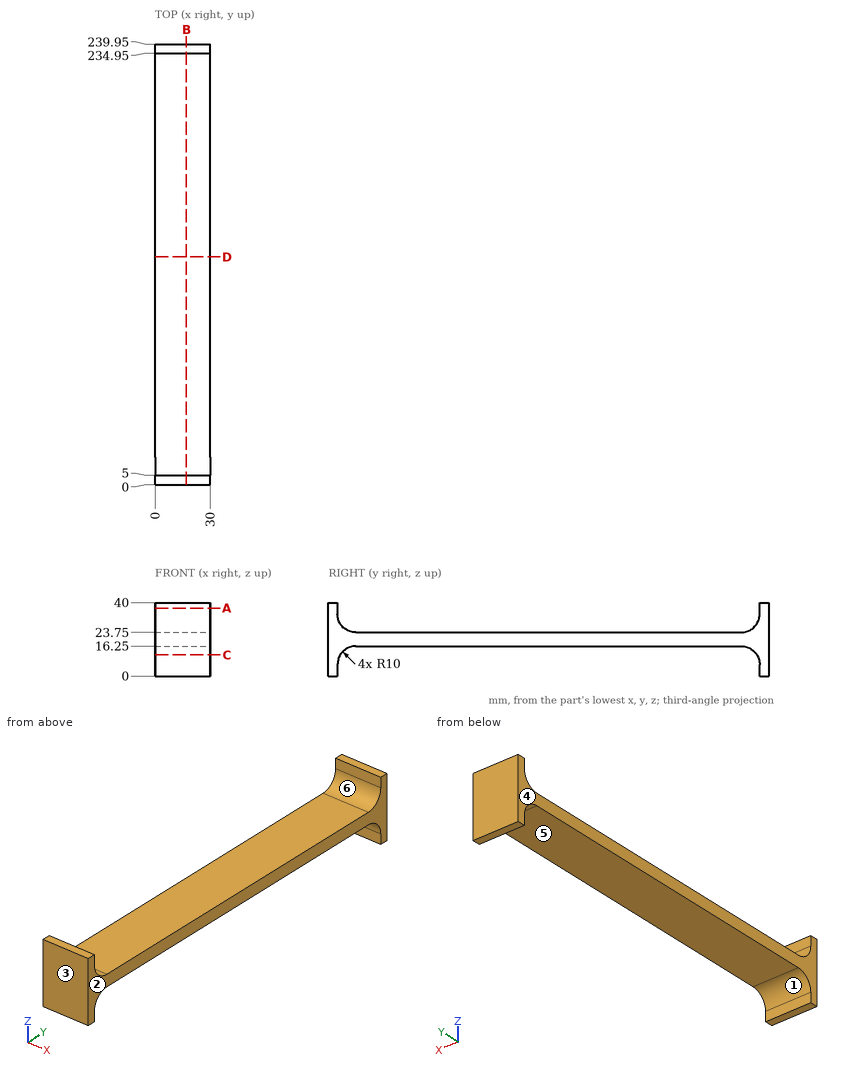
Study the drawing (mm; zero at the part's minimum x, y, z) and answer. A direction names the side the tool comes from. Coordinates: 2 decimals unless noted, no trailing zeros. Write each loop counter-clockwise with the first axis right and the second up, starting at its lowest first coordinate (ties: lowest second). Pieces come first, ordered by that corner, then holes.
Q1. Section B-B, the plane x = 17 is taken. Write down the section's boundary in (y, z), then the cut area to 3 significant figures.
Returned:
outline: (0, 0) - (5, 0) - (5, 6.25) arc R10 cw to (15, 16.25) - (224.95, 16.25) arc R10 cw to (234.95, 6.25) - (234.95, 0) - (239.95, 0) - (239.95, 40) - (234.95, 40) - (234.95, 33.75) arc R10 cw to (224.95, 23.75) - (15, 23.75) arc R10 cw to (5, 33.75) - (5, 40) - (0, 40) - close
area: 2,210 mm2
Q2. Section A-A, the plane z = 37 is taken. Write down the section's boundary in (x, y), then the cut area to 3 significant figures.
Returned:
outline: (0, 0) - (30, 0) - (30, 5) - (0, 5) - close; (0, 234.95) - (30, 234.95) - (30, 239.95) - (0, 239.95) - close
area: 300 mm2
Q3. Find the intervals of material crossed by line 1 along Y through (x, z) = (8, 36.5); line 2 along Y through (x, z) = (7.5, 7); line 3 along Z through (x, y) = (17, 168.5), in increasing order.
Returned:
line 1: y = 0 to 5, 234.95 to 239.95
line 2: y = 0 to 5.03, 234.92 to 239.95
line 3: z = 16.25 to 23.75
Q4. Which of the six approach directions +Z, -Z, +X, -X, +Y, -Y give full straight-line access (tool end or side, diameter ignored) to the marked faces 4, 5 and 6?
Returned:
face 4: +Z, -Z, -X, +Y, -Y
face 5: -Z, +X, -X
face 6: +Z, +X, -X
Q5. Section D-D, the plane y = 124 is taken. Write down the section's boundary in (x, z), then the cut area to 3 significant figures.
Returned:
outline: (0, 16.25) - (30, 16.25) - (30, 23.75) - (0, 23.75) - close
area: 225 mm2
Q6. Section C-C, the plane z = 11.5 is taken. Write down the section's boundary in (x, y).
Returned:
outline: (0, 0) - (30, 0) - (30, 6.49) - (0, 6.49) - close; (0, 233.46) - (30, 233.46) - (30, 239.95) - (0, 239.95) - close
Q7. The mould has two halves that part along Y. Classify the marked faces 1, 2 and 3: released by +Y, released by -Y, zero draft, split by the parting line, or undercut.
Returned:
face 1: undercut
face 2: zero draft
face 3: released by -Y
Q8. Given P1, Ø6, axis at y = 39.5, z = 13.5, coming from the -X side; P2, Ø9, axis at x = 17, y = 143, coming from the -Z side; P3, Ø6, axis at x = 16.5, y = 160.5, coming from the +Z side, each flat-ended and moving along its own axis, determine where each tip first touches the part or whether it passes through.
Returned:
P1: stops at x = 0
P2: stops at z = 16.25
P3: stops at z = 23.75
